Check sheet for the modelled part. Datum: model origin and axes. Units: mm. Round coordinates to 2 decimals unless told otherwise and drop trailing zeros. Write each loop counter-clockwise with the first axis right and the second up, starting at its lowest first coordinate (ties: lowest second). Pieces come first, ordered by that corner, then holes. Notation, with made-up numbers: (35, -40) -> (65, -40) arc R19 cw to (65, -31) -> close; hole circle Ø10 at (13, 31.25). An arc over 180 degrees is marked (long way). One line per item, written item: value.
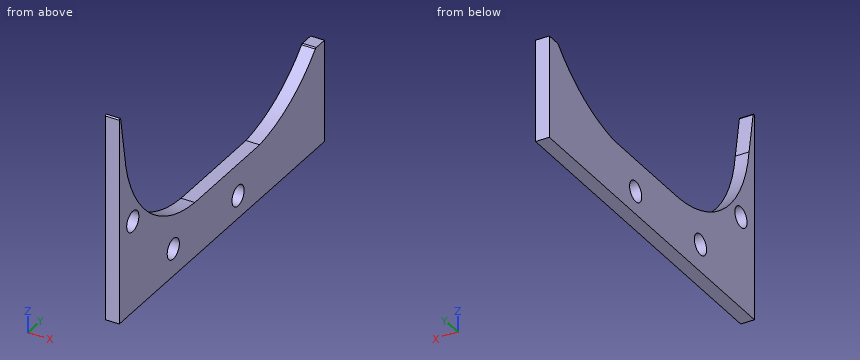
Autodesk Inventor part; units mm, degrees
ref_plane "YZ Plane" through (0, 0, 0) normal (1, 0, 0) x (0, 1, 0)
ref_plane "XZ Plane" through (0, 0, 0) normal (0, 1, 0) x (-1, 0, 0)
ref_plane "XY Plane" through (0, 0, 0) normal (0, 0, 1) x (1, 0, 0)
sketch "Sketch1" plane through (0, 0, 0) normal (1, 0, 0) x (0, 1, 0)
  line L0 (0, 0) -> (330.2, 0) construction
  line L1 (330.2, 0) -> (330.2, 304.8)
  line L2 (330.2, 304.8) -> (0, 304.8) construction
  line L3 (0, 304.8) -> (0, 0)
  line L4 (0, 0) -> (482.6, 0)
  line L5 (482.6, 0) -> (482.6, 76.2) construction
  line L6 (482.6, 76.2) -> (0, 76.2)
  line L7 (0, 76.2) -> (0, 0) construction
  circle A0 centre (330.2, 304.8) radius 76.2
  line L8 (330.2, 304.8) -> (462.0741, 141.9491) construction
  line L9 (330.2, 304.8) -> (330.2, 76.2) construction
  line L10 (330.2, 304.8) -> (403.3287, 98.2908) construction
  arc A1 (330.2, 76.2) -> (462.0741, 141.9491) centre (304.8762, 292.1181) ccw
  line L11 (330.2, 304.8) -> (254, 304.8) construction
  line L12 (254, 304.8) -> (254, 228.6) construction
  line L13 (254, 228.6) -> (330.2, 228.6) construction
  line L14 (330.2, 228.6) -> (330.2, 304.8) construction
  line L15 (254, 228.6) -> (441.325, 228.6) construction
  circle A2 centre (254, 228.6) radius 6.35
  line L16 (254, 228.6) -> (241.3, 76.2) construction
  line L17 (254, 228.6) -> (419.1, 228.6) construction
  line L18 (0, 76.2) -> (190.5, 76.2) construction
  line L19 (190.5, 76.2) -> (190.5, 228.6) construction
  line L20 (190.5, 228.6) -> (0, 228.6) construction
  line L21 (0, 228.6) -> (0, 76.2) construction
  circle A3 centre (190.5, 228.6) radius 6.35
  line L22 (190.5, 228.6) -> (76.0017, 114.1017) construction
  line L23 (190.5, 228.6) -> (352.425, 228.6) construction
  line L24 (190.5, 228.6) -> (12.7, 228.6) construction
  arc A4 (12.7, 228.6) -> (190.5, 76.2) centre (184.0395, 248.5794) ccw
  line L25 (12.7, 228.6) -> (0, 304.8)
  line L26 (462.0741, 141.9491) -> (482.6, 141.9491)
  line L27 (482.6, 141.9491) -> (482.6, 0)
  line L28 (330.2, 76.2) -> (177.5789, 76.2)
  dimension "d0" = 330.2
  dimension "d1" = 304.8
  dimension "d2" = 482.6
  dimension "d3" = 76.2
  dimension "d4" = 152.4
  dimension "d5" = 209.55
  dimension "d9" = 228.6
  dimension "d13" = 219.075
  dimension "d16" = 39
  dimension "d17" = 19.5
  dimension "d19" = 76.2
  dimension "d20" = 76.2
  dimension "d25" = 12.7
  dimension "d39" = 190.5
  dimension "d40" = 152.4
  dimension "d41" = 12.7
  dimension "d42" = 161.925
  dimension "d43" = 135
  dimension "d44" = 177.8
extrude "Extrusion1" add sketch "Sketch1" along normal blind 19.05 contours L4 L3 L6 A4 L1 | L1 L6 L27 L4 | A1 L26 L27 L6 | A4 L6 | L3 L25 A4 L6
fillet "Fillet1" radius 1.5875 1 edges at (9.525, 0, 304.8)
fillet "Fillet2" radius 3.175 1 edges at (9.525, 462.0741, 141.9491)
sketch "Sketch2" plane through (19.05, 0, 0) normal (1, 0, 0) x (0, 0, -1)
  line L0 (0, 482.6) -> (0, 0)
  line L1 (0, 0) -> (-127, 0)
  line L2 (-127, 0) -> (-127, 31.75)
  line L3 (-127, 31.75) -> (0, 31.75)
  line L4 (0, 31.75) -> (0, 0)
  circle A0 centre (-127, 31.75) radius 25.4
  line L5 (0, 0) -> (-285.6186, 0)
  line L6 (0, 0) -> (-38.1, 0)
  line L7 (-38.1, 0) -> (-38.1, 127)
  line L8 (0, 127) -> (0, 0)
  line L9 (0, 127) -> (-38.1, 127)
  circle A1 centre (-38.1, 127) radius 50.8
  line L10 (0, 0) -> (-31.75, 0)
  line L11 (-31.75, 0) -> (-31.75, 279.4)
  line L12 (-31.75, 279.4) -> (0, 279.4)
  line L13 (0, 279.4) -> (0, 0)
  circle A2 centre (-31.75, 279.4) radius 50.8
  dimension "d49" = 127
  dimension "d50" = 31.75
  dimension "d51" = 50.8
  dimension "d52" = 38.1
  dimension "d53" = 101.6
  dimension "d54" = 279.4
  dimension "d55" = 101.6
  dimension "d56" = 31.75
  dimension "d57" = 127
hole "Hole1" at (19.05, 31.75, 127) at (19.05, 127, 38.1) at (19.05, 279.4, 31.75) direction (-1, 0, 0) diameter 28.575 end through all
properties part number "New Shooter Curve"
Item 1: Sectioned sample at C-C on z = 127. Enter the section's corners in (x, y).
Answer:
outline: (0, 0) -> (19.05, 0) -> (19.05, 17.46) -> (0, 17.46) -> close; (0, 46.04) -> (19.05, 46.04) -> (19.05, 61.67) -> (0, 61.67) -> close; (0, 446.29) -> (19.05, 446.29) -> (19.05, 482.6) -> (0, 482.6) -> close
Item 2: Sectioned sample at B-B on y = 279.4. Enter the section's corners in (x, z).
Answer:
outline: (0, 0) -> (19.05, 0) -> (19.05, 17.46) -> (0, 17.46) -> close; (0, 46.04) -> (19.05, 46.04) -> (19.05, 76.2) -> (0, 76.2) -> close
Item 3: Sectioned sample at A-A on x = 7.5. Count the separate pieces of the cut face and the enclosed holes in it, and give its area (3 significant figures).
Answer:
separate pieces: 1
enclosed holes: 3
area: 47,800 mm^2
Item 4: Depth check by flat-ended pin: P1, Ø4, axis at x = 10, y = 392, coming from the +Z side; P2, Ø2, axis at x = 14, y = 133.5, coming from the +Z side; P3, Ø23, axis at y = 31.75, z = 127, coming from the -X side. Enter the tip coordinate at first touch or a pass-through.
Answer:
P1: stops at z = 93.83
P2: stops at z = 83.96
P3: passes through
Item 5: Thickness scan on line 1 (Z direction, x = 8, y = 279.4); line 2 (Y direction, x = 8.5, z = 38.1); line 3 (Z direction, x = 5.5, y = 316.5). Record the ranges inside material, lowest first.
Answer:
line 1: z = 0 to 17.46, 46.04 to 76.2
line 2: y = 0 to 112.71, 141.29 to 266.6, 292.2 to 482.6
line 3: z = 0 to 76.2
Item 6: Sectioned sample at D-D on z = 39.5. Enter the section's corners in (x, y).
Answer:
outline: (0, 0) -> (19.05, 0) -> (19.05, 112.78) -> (0, 112.78) -> close; (0, 141.22) -> (19.05, 141.22) -> (19.05, 267.4) -> (0, 267.4) -> close; (0, 291.4) -> (19.05, 291.4) -> (19.05, 482.6) -> (0, 482.6) -> close
